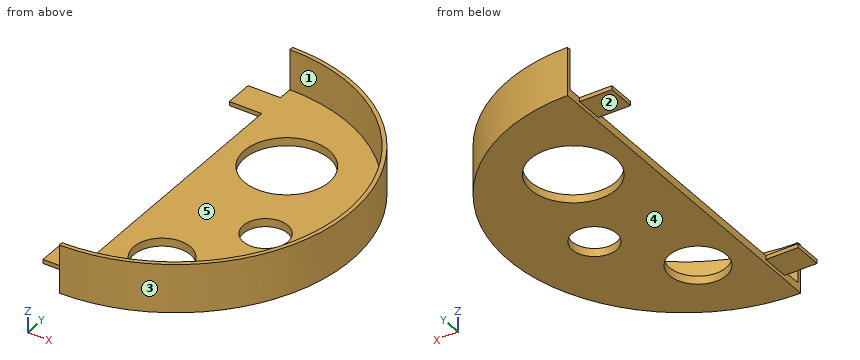
from build123d import *

# Parameters (mm, degrees)
F1_DEPTH = 12
F2_R     = 42.5
F3_DEPTH = 10
F4_R     = 10.5
F4_R_2   = 5.5
F4_R_3   = 7
F5_DEPTH = 2.001
F6_W     = 7
F6_H     = 1
F7_DEPTH = 8


with BuildPart() as f1:
    # F0 (on Top) → F1 (new body)
    with BuildSketch(Plane.XY):
        with BuildLine():
            Line((0, 43.5), (0, -43.5))
            ThreePointArc((0, -43.5), (43.5, 0), (0, 43.5))
        make_face()
    extrude(amount=F1_DEPTH)

    # F2 (on face) → F3 (cut)
    with BuildSketch(Plane.XY.offset(12)):
        Circle(F2_R)
    extrude(amount=-F3_DEPTH, mode=Mode.SUBTRACT)

    # F4 (on face) → F5 (cut, through all)
    with BuildSketch(Plane.XY.offset(2)):
        with Locations((-15, 18.734994)):
            Circle(F4_R)
        with Locations((-25, -4.265006)):
            Circle(F4_R_2)
        with Locations((-12, -23.265006)):
            Circle(F4_R_3)
        with Locations((15, 18.734994)):
            Circle(F4_R)
        with Locations((25, -4.265006)):
            Circle(F4_R_2)
        with Locations((12, -23.265006)):
            Circle(F4_R_3)
    extrude(amount=-F5_DEPTH, mode=Mode.SUBTRACT)

    # F6 (on face) → F7 (join)
    with BuildSketch(Plane(origin=(0, 0, 0), x_dir=(0, -1, 0), z_dir=(-1, 0, 0))):
        with Locations((-35.5, 1.5)):
            Rectangle(F6_W, F6_H)
        with Locations((34, 1.5)):
            Rectangle(F6_W, F6_H)
    extrude(amount=F7_DEPTH)


solid = f1.part
Part model, mm, in its own coordinate system. Face numbers are marked on the shaded views. A direction names the side the tool comes from. Coordinates: 2 decimals unless noted, no trailing zeros. Write each loop counter-clockwise with the first axis right and the second up, starting at its lowest first coordinate (ties: lowest second). Pieces come first, ordered by that corner, then holes. Notation, with made-up numbers: M 62,53 L 112,53 A25 ccw 112,85 Z; hole C 80.25,-32 d4. An arc over 180 degrees is marked long. Return JSON: item names as keys, results as strings.
1. Saw through at B-B, the plane y = 28. Write the cut outline in (x, z).
Determined:
{"outline": "M 0,0 L 10.06,0 L 10.06,2 L 0,2 Z; M 19.94,0 L 33.29,0 L 33.29,12 L 31.97,12 L 31.97,2 L 19.94,2 Z"}
2. Saw through at C-C, the plane z = 10.75. Write the cut outline in (x, y), then the cut area to 3 significant figures.
Determined:
{"outline": "M 0,-43.5 A43.5 ccw 0,43.5 L 0,42.5 A42.5 cw 0,-42.5 Z", "area": "135 mm²"}
3. 3-axis set-ups, long thin cutter, end or side, ignore diameter. For the marked faces 1 and 2: which of +Z, -Z, +X, -X, +Y, -Y reach the whole face in a straight line?
Determined:
{"face 1": "+Z, -X", "face 2": "-Z, -X, +Y, -Y"}
4. Saw through at D-D, the plane y = -1. Write the cut outline in (x, z), then the cut area to 3 significant figures.
Determined:
{"outline": "M 0,0 L 20.57,0 L 20.57,2 L 0,2 Z; M 29.43,0 L 43.49,0 L 43.49,12 L 42.49,12 L 42.49,2 L 29.43,2 Z", "area": "79.3 mm²"}
5. Flat gauge pins, fed straight in: pin 1 Ø6 at (x, z) = (15.5, 6) entering from +Y; pin 2 Ø0.5 at (x, z) = (-4, 1.5) entering from +Y; pin 3 Ø6 at (y, z) = (-2, 9) entering from -X. Where does each tip first touch, or does it go through?
Determined:
{"pin 1": "y = 41.67", "pin 2": "y = 39", "pin 3": "x = 42.2"}
6. Saw through at A-A, the plane x = 12. Write the cut outline in (y, z) (3 decimals), then the cut area to 3 significant figures.
Determined:
{"outline": "M -41.812,0 L -30.265,0 L -30.265,2 L -40.771,2 L -40.771,12 L -41.812,12 Z; M -16.265,0 L 8.673,0 L 8.673,2 L -16.265,2 Z; M 28.797,0 L 41.812,0 L 41.812,12 L 40.771,12 L 40.771,2 L 28.797,2 Z", "area": "120 mm²"}
7. Pull direction Y, two halves, no side cores. Call the marked faces 3, 4 and 5: pulls with the +Y half, pulls with the -Y half, needs draft (parallel to the pull), parting line crosses it, or undercut.
Determined:
{"face 3": "parting line crosses it", "face 4": "needs draft", "face 5": "undercut"}
8. Probe L1, parallel to Y at x = 21.5, z = 1.25; L2, parallel to Y at x = 12, z = 1.55 (3 decimals); L3, parallel to Z at x = 15, y = 4.5. List the from-to ranges inside material, lowest first.
Determined:
{"L1": "-37.82 to -8.51, -0.02 to 10.49, 26.98 to 37.82", "L2": "-41.812 to -30.265, -16.265 to 8.673, 28.797 to 41.812", "L3": "0 to 2"}
